from build123d import *

# Parameters (mm, degrees)
F1_DEPTH = 666.75
F2_R     = 3.96875
F3_DEPTH = 50.8
F4_R     = 3.175
F5_DEPTH = 50.8
F7_DEPTH = 25.4
F8_DEPTH = 25.4


with BuildPart() as f1:
    # F0 (on Top) → F1 (new body)
    with BuildSketch(Plane.XY):
        Polygon((-25.4, 12.7), (-25.4, -12.7), (-22.225, -12.7), (-22.225, 9.525), (22.225, 9.525), (22.225, -12.7), (25.4, -12.7), (25.4, 12.7), align=None)
    extrude(amount=F1_DEPTH)

    # F2 (on face) → F3 (cut, through all)
    with BuildSketch(Plane.YZ.offset(25.4)):
        with Locations((0, 16.51)):
            Circle(F2_R)
        with Locations((0, 54.61)):
            Circle(F2_R)
    extrude(amount=-F3_DEPTH, mode=Mode.SUBTRACT)

    # F4 (on face) → F5 (cut, through all)
    with BuildSketch(Plane.YZ.offset(25.4)):
        with Locations((-4.7625, 658.7236)):
            Circle(F4_R)
    extrude(amount=-F5_DEPTH, mode=Mode.SUBTRACT)

    # F6 (on face) → F7 (cut)
    with BuildSketch(Plane(origin=(0, 12.7, 0), x_dir=(-1, 0, 0), z_dir=(0, 1, 0))):
        with BuildLine():
            Line((22.225, 666.75), (-22.225, 666.75))
            Line((-22.225, 666.75), (-22.225, 608.0125))
            ThreePointArc((-22.225, 608.0125), (-20.830096, 604.644904), (-17.4625, 603.25))
            Line((-17.4625, 603.25), (17.4625, 603.25))
            ThreePointArc((17.4625, 603.25), (20.830096, 604.644904), (22.225, 608.0125))
            Line((22.225, 608.0125), (22.225, 666.75))
        make_face()
    extrude(amount=-F7_DEPTH, mode=Mode.SUBTRACT)

    # F0 (on Top) → F8 (join)
    with BuildSketch(Plane.XY):
        Polygon((-25.4, 12.7), (-25.4, -12.7), (-22.225, -12.7), (-22.225, 9.525), (22.225, 9.525), (22.225, -12.7), (25.4, -12.7), (25.4, 12.7), align=None)
    extrude(amount=F8_DEPTH)


solid = f1.part
For this review, take the finished solid that the model builds, in its own axes (mm). Give positions to 0.01 mm unless a question says otherwise; leave off trailing zeros. Loops run counter-clockwise (first coordinate to the right, second up) from the corner with the lowest first, then second, coordinate; pieces in that order, holes last.
Item 1: For line 1 along X through (y, z) = (-11.5, 86) (3 decimals); line 2 along Z through (x, y) = (22.9, 0); line 3 along Y through (x, z) = (-1, 404) (3 decimals), list the stretches that pass through material, from the lowest coordinate up.
Item 2: Take a section at A-A, the plane z = 398.5. State the section outline as (x, y) points (3 decimals), and give its area (3 significant figures).
Item 3: Insertion check: pin 1 (6 mm diameter, centred on x = 1.5, y = 4.5, fed in from -Z); pin 2 (13.5 mm diameter, centred on x = 4.5, z = 313.5, fed in from -Y) (3 decimals); pin 3 (1 mm diameter, centred on x = 5.5, y = 10.5, fed in from +Z). Each pin has a flat end and moves straight along its axis. Give the tip position at first contact, or say it passes through.
Item 4: Take a section at B-B, the plane x = -2.5. State the section outline as (y, z) points (3 decimals).
Item 5: Draft analysis for pull direction X (two halves, no side actions). For faces 1 (the flat face through (22.225, 0, 338)), 2 (the flat face through (0, 12.7, 329)), 3 (the flat face through (-25.4, 0, 329)), 4 (the flat face through (0, 9.525, 300)), state which applies: +X half, -X half, draft (parallel to the pull), parting line (faces both ways), or undercut.
Calculated:
1. line 1: x = -25.4 to -22.225, 22.225 to 25.4
1. line 2: z = 0 to 50.64, 58.58 to 666.75
1. line 3: y = 9.525 to 12.7
2. outline: (-25.4, -12.7) - (-22.225, -12.7) - (-22.225, 9.525) - (22.225, 9.525) - (22.225, -12.7) - (25.4, -12.7) - (25.4, 12.7) - (-25.4, 12.7) - close
2. area: 302 mm2
3. pin 1: passes through
3. pin 2: stops at y = 9.525
3. pin 3: stops at z = 603.25
4. outline: (9.525, 0) - (12.7, 0) - (12.7, 603.25) - (9.525, 603.25) - close
5. face 1: undercut
5. face 2: draft
5. face 3: -X half
5. face 4: undercut
